from build123d import *

# Parameters (mm, degrees)
SKETCH1_R                                      = 29.692527183
SKETCH1_R_2                                    = 22.692527183
SKETCH1_R_3                                    = 19.692527183
SKETCH1_R_4                                    = 16.692527183
BOSS_EXTRUDE1_DEPTH                            = 5
SKETCH9_W                                      = 27.5
SKETCH9_H                                      = 28
BOSS_EXTRUDE2_DEPTH                            = 7.5
SKETCH10_W                                     = 23.5
SKETCH10_H                                     = 25.45
CUT_EXTRUDE1_DEPTH                             = 6.1
SKETCH12_W                                     = 12
SKETCH12_H                                     = 11
CUT_EXTRUDE2_DEPTH                             = 3
SKETCH11_W                                     = 13
SKETCH11_H                                     = 9.717675131
CUT_EXTRUDE3_DEPTH                             = 4.947760199
CSK_FOR_M3_FLAT_HEAD_MACHINE_SCREW1_AT_2_COUNT = 2
CSK_FOR_M3_FLAT_HEAD_MACHINE_SCREW1_AT_2_PITCH = 27.84943902
CSK_FOR_M3_FLAT_HEAD_MACHINE_SCREW1_AT_3_COUNT = 2
CSK_FOR_M3_FLAT_HEAD_MACHINE_SCREW1_AT_3_PITCH = 27.84943902
CSK_FOR_M3_FLAT_HEAD_MACHINE_SCREW1_AT_4_COUNT = 2
CSK_FOR_M3_FLAT_HEAD_MACHINE_SCREW1_AT_4_PITCH = 39.385054366
SPLIT1_START                                   = -28
SPLIT1_DEPTH                                   = 28
SPLIT1_2_OUTLINE_W                             = 23.5
SPLIT1_2_OUTLINE_H                             = 0.6
SPLIT1_2_DEPTH                                 = 2.602239801
SPLIT1_START_2                                 = 5.5
SPLIT1_3_OUTLINE_W                             = 27.5
SPLIT1_3_OUTLINE_H                             = 28
SPLIT1_3_DEPTH                                 = 2


# Read off the part's stored shape, not the designer's step: Split1
with BuildPart() as part:
    # Sketch1 → Boss-Extrude1 (new body)
    # profile 1 of 4: a face of its own
    with BuildSketch(Plane(origin=(0, 0, 0), x_dir=(-1, 0, 0), z_dir=(0, 0, 1))):
        with Locations(Location((0, 0, 0), (0, 0, 180))):
            Circle(SKETCH1_R)
        Circle(SKETCH1_R_2, mode=Mode.SUBTRACT)
    # profile 2 of 4: a face of its own
    with BuildSketch(Plane(origin=(0, 0, 0), x_dir=(-1, 0, 0), z_dir=(0, 0, 1))):
        Circle(SKETCH1_R_2)
        Circle(SKETCH1_R_3, mode=Mode.SUBTRACT)
    # profile 3 of 4: a face of its own
    with BuildSketch(Plane(origin=(0, 0, 0), x_dir=(-1, 0, 0), z_dir=(0, 0, 1))):
        Circle(SKETCH1_R_3)
        Circle(SKETCH1_R_4, mode=Mode.SUBTRACT)
    # profile 4 of 4: a face of its own
    with BuildSketch(Plane(origin=(0, 0, 0), x_dir=(-1, 0, 0), z_dir=(0, 0, 1))):
        with BuildLine():
            Line((14.058465911, 9), (-14.058465911, 9))
            ThreePointArc((-14.058465911, 9), (-16.692527183, 0), (-14.058465911, -9))
            Line((-14.058465911, -9), (14.058465911, -9))
            ThreePointArc((14.058465911, -9), (16.020483578, -4.688770595), (16.692527183, 0))
            ThreePointArc((16.692527183, 0), (16.020483578, 4.688770595), (14.058465911, 9))
        make_face()
    extrude(amount=BOSS_EXTRUDE1_DEPTH)

    # Sketch9 → Boss-Extrude2 (add, symmetric)
    with BuildSketch(Plane(origin=(0, 0, 0), x_dir=(1, 0, 0), z_dir=(0, 1, 0))):
        with Locations((5.7, 14)):
            Rectangle(SKETCH9_W, SKETCH9_H)
    extrude(amount=BOSS_EXTRUDE2_DEPTH, both=True)

    # Sketch10 → Cut-Extrude1 (cut, symmetric)
    with BuildSketch(Plane(origin=(0, 0, 0), x_dir=(1, 0, 0), z_dir=(0, 1, 0))):
        with Locations((5.7, 12.672760199)):
            Rectangle(SKETCH10_W, SKETCH10_H)
    extrude(amount=CUT_EXTRUDE1_DEPTH, both=True, mode=Mode.SUBTRACT)

    # Sketch12 → Cut-Extrude2 (cut)
    with BuildSketch(Plane.XY.offset(-28)):
        with Locations((1.95, 0)):
            Rectangle(SKETCH12_W, SKETCH12_H)
    extrude(amount=CUT_EXTRUDE2_DEPTH, mode=Mode.SUBTRACT)

    # Sketch11 → Cut-Extrude3 (cut)
    with BuildSketch(Plane.XY.offset(5)):
        with Locations((-1.55, -0.433824782)):
            Rectangle(SKETCH11_W, SKETCH11_H)
    extrude(amount=-CUT_EXTRUDE3_DEPTH, mode=Mode.SUBTRACT)

    # Sketch13 → CSK for M3 Flat Head Machine Screw1 (revolve, cut)
    with BuildSketch(Plane.YZ.offset(-19.692527183)):
        Polygon((0, 0), (0, 13.021463052), (1.7, 12), (1.7, 1.95), (3.65, 0), align=None)
    csk_for_m3_flat_head_machine_screw1 = revolve(axis=Axis((-19.692527183, 0, -6.35), (0, 0, 1)), mode=Mode.SUBTRACT)

    # CSK for M3 Flat Head Machine Screw1 at 2: CSK for M3 Flat Head Machine Screw1 ×2
    with Locations(*[Vector(0.7071067811865476, -0.7071067811865475, 0) * (i * CSK_FOR_M3_FLAT_HEAD_MACHINE_SCREW1_AT_2_PITCH) for i in range(1, CSK_FOR_M3_FLAT_HEAD_MACHINE_SCREW1_AT_2_COUNT)]):
        add(csk_for_m3_flat_head_machine_screw1, mode=Mode.SUBTRACT)

    # CSK for M3 Flat Head Machine Screw1 at 3: CSK for M3 Flat Head Machine Screw1 ×2
    with Locations(*[Vector(0.7071067811865476, 0.7071067811865475, 0) * (i * CSK_FOR_M3_FLAT_HEAD_MACHINE_SCREW1_AT_3_PITCH) for i in range(1, CSK_FOR_M3_FLAT_HEAD_MACHINE_SCREW1_AT_3_COUNT)]):
        add(csk_for_m3_flat_head_machine_screw1, mode=Mode.SUBTRACT)

    # CSK for M3 Flat Head Machine Screw1 at 4: CSK for M3 Flat Head Machine Screw1 ×2
    with Locations(*[(i * CSK_FOR_M3_FLAT_HEAD_MACHINE_SCREW1_AT_4_PITCH, 0, 0) for i in range(1, CSK_FOR_M3_FLAT_HEAD_MACHINE_SCREW1_AT_4_COUNT)]):
        add(csk_for_m3_flat_head_machine_screw1, mode=Mode.SUBTRACT)

    # Split1 3 outline → Split1 3 (cut)
    with BuildSketch(Plane(origin=(0, 0, 0), x_dir=(1, 0, 0), z_dir=(0, 1, 0)).offset(SPLIT1_START_2)):
        with Locations((5.7, 14)):
            Rectangle(SPLIT1_3_OUTLINE_W, SPLIT1_3_OUTLINE_H)
    extrude(amount=SPLIT1_3_DEPTH, mode=Mode.SUBTRACT)


with BuildPart() as body_2:
    # Split1 outline → Split1 (new body)
    with BuildSketch(Plane.XY.offset(SPLIT1_START)):
        Polygon((-8.05, 5.5), (-6.05, 5.5), (-6.05, 6.1), (17.45, 6.1), (17.45, 5.5), (19.45, 5.5), (19.45, 7.5), (-8.05, 7.5), align=None)
    extrude(amount=SPLIT1_DEPTH)

    # Split1 2 outline → Split1 2 (add)
    with BuildSketch(Plane.XY.offset(SPLIT1_START)):
        with Locations((5.7, 5.8)):
            Rectangle(SPLIT1_2_OUTLINE_W, SPLIT1_2_OUTLINE_H)
    extrude(amount=SPLIT1_2_DEPTH)


solid = body_2.part
Geometry check sheet. Reference: the model listing, model coordinates, mm. Give positions to 0.01 mm unless a question says otherwise; leave off trailing zeros. Loops run counter-clockwise (first coordinate to the right, second up) from the corner with the lowest first, then second, coordinate; pieces in that order, holes last. Notation, with made-up numbers: (81.25, 10.25) -> (88.25, 10.25) arc R23 ccw to (88.25, 19.25) -> close; hole circle Ø1 at (42.5, -1.5). An arc over 180 degrees is marked (long way). Answer in a Markdown table with one row per item. Add a question column.
1) Cross-section at B-B on x = -1. Record the boundary of the cut face in (y, z), and give its area (3 significant figures).
2) Draft check along X on faces 1 (the face through (6, 6.1, -13)), 2 (the face through (6, 5.5, -27)), 3 (the face through (19.45, 6, -14)), 4 (the face through (-8.05, 7, -14)). Enter one of: pulls with the +X half, pulls with the -X half, needs draft (parallel to the pull), parting line crosses it, or undercut.
3) Cross-section at A-A on z = -15.25. Record the boundary of the cut face in (x, y), and give its area (3 significant figures).
4) Material ranges on probe 1 along X at (y, z) = (5.8, -24.75); probe 2 along Y at (x, z) = (3, -3.5); probe 3 along Z at (x, y) = (0.25, 5.7), recorded low to high. Write a range as from..to.
5) Gauge pin test, flat ends, axial feed: P1, Ø3, axis at x = 9.5, z = -18.5, coming from the -Y side; P2, Ø0.7, axis at x = 0, y = 6, coming from the +Z side. Record the tip position at first contact, or that the pin passes through.
Outcome:
| question | item | result |
|---|---|---|
| 1 | outline | (5.5, -28) -> (7.5, -28) -> (7.5, 0) -> (6.1, 0) -> (6.1, -25.4) -> (5.5, -25.4) -> close |
| 1 | area | 40.8 mm^2 |
| 2 | face 1 | undercut |
| 2 | face 2 | needs draft |
| 2 | face 3 | pulls with the +X half |
| 2 | face 4 | pulls with the -X half |
| 3 | outline | (-8.05, 5.5) -> (-6.05, 5.5) -> (-6.05, 6.1) -> (17.45, 6.1) -> (17.45, 5.5) -> (19.45, 5.5) -> (19.45, 7.5) -> (-8.05, 7.5) -> close |
| 3 | area | 40.9 mm^2 |
| 4 | probe 1 | x = -8.05..-6.05, 17.45..19.45 |
| 4 | probe 2 | y = 6.1..7.5 |
| 4 | probe 3 | z = -28..-25.4 |
| 5 | P1 | stops at y = 6.1 |
| 5 | P2 | stops at z = 0 |
